```python
from build123d import *

# Parameters (mm, degrees)
SKETCH1_W           = 482.6
SKETCH1_H           = 304.8
BOSS_EXTRUDE1_DEPTH = 12.7
BOSS_EXTRUDE2_DEPTH = 6.35
SKETCH3_R           = 1.5875
CUT_EXTRUDE1_DEPTH  = 507.449822292
SKETCH4_W           = 6.35
SKETCH4_H           = 12.7
BOSS_EXTRUDE3_DEPTH = 292.1
SKETCH5_W           = 12.7
SKETCH5_H           = 19.05
BOSS_EXTRUDE4_DEPTH = 6.35
CUT_EXTRUDE2_START  = 6.35
CUT_EXTRUDE2_DEPTH  = 25.4
CUT_EXTRUDE3_START  = -488.95
CUT_EXTRUDE3_DEPTH  = 25.4
BOSS_EXTRUDE5_START = -2.54
BOSS_EXTRUDE5_DEPTH = 7.62
SKETCH13_W          = 304.8
SKETCH13_H          = 12.7
CUT_EXTRUDE4_DEPTH  = 519.566054134
SKETCH17_W          = 369.208963073
SKETCH17_H          = 308.023191689
CUT_EXTRUDE7_DEPTH  = 291.854955261


with BuildPart() as part:
    # Sketch1 → Boss-Extrude1 (new body)
    with BuildSketch(Plane(origin=(0, 0, 0), x_dir=(1, 0, 0), z_dir=(0, 1, 0))):
        Rectangle(SKETCH1_W, SKETCH1_H)
    extrude(amount=BOSS_EXTRUDE1_DEPTH)

    # Sketch2 → Boss-Extrude2 (add)
    with BuildSketch(Plane(origin=(0, 12.7, 0), x_dir=(1, 0, 0), z_dir=(0, 1, 0))):
        Polygon((-241.3, 152.4), (-228.6, 152.4), (228.6, 152.4), (241.3, 152.4), (241.3, -152.4), (228.6, -152.4), (228.6, 28.575), (-228.6, 28.575), (-228.6, -152.4), (-241.3, -152.4), align=None)
    extrude(amount=BOSS_EXTRUDE2_DEPTH)

    # Sketch3 → Cut-Extrude1 (cut, through all)
    with BuildSketch(Plane.ZY.offset(241.3)):
        with Locations((149.225, 15.875)):
            Circle(SKETCH3_R)
    extrude(amount=-CUT_EXTRUDE1_DEPTH, mode=Mode.SUBTRACT)

    # Sketch4 → Boss-Extrude3 (add)
    with BuildSketch(Plane.XY.offset(152.4)):
        with Locations((-244.475, 6.35)):
            Rectangle(SKETCH4_W, SKETCH4_H)
    boss_extrude3 = extrude(amount=-BOSS_EXTRUDE3_DEPTH)

    # Sketch5 → Boss-Extrude4 (add)
    with BuildSketch(Plane.ZY.offset(241.3)):
        with Locations((-146.05, 9.525)):
            Rectangle(SKETCH5_W, SKETCH5_H)
    boss_extrude4 = extrude(amount=BOSS_EXTRUDE4_DEPTH)

    # Mirror1: Boss-Extrude3, Boss-Extrude4 across plane
    add(boss_extrude3.mirror(Plane(origin=(0, 0, 0), x_dir=(0, 0, 1), z_dir=(1, 0, 0))))
    add(boss_extrude4.mirror(Plane(origin=(0, 0, 0), x_dir=(0, 0, 1), z_dir=(1, 0, 0))))

    # Sketch6 → Cut-Extrude2 (cut)
    with BuildSketch(Plane.ZY.offset(241.3).offset(CUT_EXTRUDE2_START)):
        with BuildLine():
            Line((147.32, 2.54), (128.27, 2.54))
            ThreePointArc((128.27, 2.54), (124.46, 6.35), (128.27, 10.16))
            Line((128.27, 10.16), (147.32, 10.16))
            ThreePointArc((147.32, 10.16), (151.13, 6.35), (147.32, 2.54))
        make_face()
    extrude(amount=-CUT_EXTRUDE2_DEPTH, mode=Mode.SUBTRACT)

    # Sketch6<2> → Cut-Extrude3 (cut)
    with BuildSketch(Plane.ZY.offset(241.3).offset(CUT_EXTRUDE3_START)):
        with BuildLine():
            Line((147.32, 2.54), (128.27, 2.54))
            ThreePointArc((128.27, 2.54), (124.46, 6.35), (128.27, 10.16))
            Line((128.27, 10.16), (147.32, 10.16))
            ThreePointArc((147.32, 10.16), (151.13, 6.35), (147.32, 2.54))
        make_face()
    extrude(amount=CUT_EXTRUDE3_DEPTH, mode=Mode.SUBTRACT)

    # Sketch11 → Boss-Extrude5 (add)
    with BuildSketch(Plane.XZ.offset(BOSS_EXTRUDE5_START)):
        Polygon((-247.65, 124.46), (-222.25, 124.46), (-222.25, 140.97), align=None)
    boss_extrude5 = extrude(amount=-BOSS_EXTRUDE5_DEPTH)

    # Mirror2: Boss-Extrude5 across plane
    add(boss_extrude5.mirror(Plane(origin=(0, 0, 0), x_dir=(0, 0, 1), z_dir=(1, 0, 0))))

    # Sketch13 → Cut-Extrude4 (cut, through all)
    with BuildSketch(Plane.ZY.offset(247.65)):
        with Locations((0, 6.35)):
            Rectangle(SKETCH13_W, SKETCH13_H)
    extrude(amount=-CUT_EXTRUDE4_DEPTH, mode=Mode.SUBTRACT)

    # Sketch17 → Cut-Extrude7 (cut, through all)
    with BuildSketch(Plane(origin=(0, 19.05, 0), x_dir=(1, 0, 0), z_dir=(0, 1, 0))):
        with Locations((-89.354481537, -1.611595845)):
            Rectangle(SKETCH17_W, SKETCH17_H)
    extrude(amount=-CUT_EXTRUDE7_DEPTH, mode=Mode.SUBTRACT)


solid = part.part
```
Read the model definition and answer for the solid it produces. Units are mm, in the model's axes. A direction names the side the tool comes from. Coordinates: 2 decimals unless noted, no trailing zeros. Loops run counter-clockwise (first coordinate to the right, second up) from the corner with the lowest first, then second, coordinate; pieces in that order, holes last. Notation, with made-up numbers: (-9, 8.5) -> (10, 8.5) arc R22 cw to (10, 37.5) -> close; hole circle Ø10 at (-17, 76.25). An arc over 180 degrees is marked (long way). Return JSON: item names as keys, results as strings.
Item 1: Find section A-A (x = 203.5). Determine the outline of the cut face in (y, z) (3 decimals), plus the area to 3 significant figures.
Answers:
{"outline": "(12.7, -152.4) -> (19.05, -152.4) -> (19.05, -28.575) -> (12.7, -28.575) -> close", "area": "786 mm2"}
Item 2: Flat-ended cylindrical pins translate along their axes: P1, Ø1.9, axis at x = 157.5, y = 15, coming from the +Z side (3 decimals); P2, Ø1, axis at y = 15, z = -79.5, coming from the +X side. Find the tip coordinate at first contact, or state that the pin passes through.
Answers:
{"P1": "stops at z = -28.575", "P2": "stops at x = 241.3"}
Item 3: For faces 1 (the flat face through (163, 16, -28.575)), 2 (the flat face through (244, 16, -139.7)), 3 (the flat face through (170, 19.05, -70)), determine the directions among +Z, -Z, +X, -X, +Y, -Y from which every point of the face is accessible in a straight line to the end or side of a thin tool.
Answers:
{"face 1": "+Z, -X, +Y, -Y", "face 2": "+Z, +X, +Y, -Y", "face 3": "+Z, -Z, +X, -X, +Y"}
Item 4: Find section B-B (z = -78.5). Determine the outline of the cut face in (x, y).
Answers:
{"outline": "(95.25, 12.7) -> (241.3, 12.7) -> (241.3, 19.05) -> (95.25, 19.05) -> close"}
Item 5: Find the intervals of material crossed by probe 1 along Z at (x, y) = (207, 15.5) (3 decimals); probe 2 along X at (y, z) = (18, -124); probe 3 along X at (y, z) = (16.25, 2), in increasing order.
Answers:
{"probe 1": "z = -152.4 to -28.575", "probe 2": "x = 95.25 to 241.3", "probe 3": "x = 228.6 to 241.3"}
